The listing builds one solid part. Answer for the finished solid, in the listing's coordinates (mm). Face numbers are marked on the shaded views. A direction names the side the tool comes from. Give positions to 0.01 mm unless a question says otherwise; leave off trailing zeros. Order: outer loops, then holes, each group sorted by start corner. A loop starts at its lowest first (then second) coordinate and runs counter-clockwise, first axis right, second up.
```python
from build123d import *

# Parameters (mm, degrees)
BOSS_EXTRUDE1_DEPTH = 35
SKETCH2_R           = 2
CUT_EXTRUDE1_DEPTH  = 83.927679336
CUT_EXTRUDE2_REACH  = 64.699
SKETCH3_R           = 4


with BuildPart() as part:
    # Sketch1 → Boss-Extrude1 (new body)
    with BuildSketch(Plane(origin=(0, 0, 0), x_dir=(1, 0, 0), z_dir=(0, 1, 0))):
        with BuildLine():
            Line((-36, 30), (-36, 0))
            ThreePointArc((-36, 0), (-0.776670285, -35.991621015), (35.966487959, -1.552979031))
            Line((35.966487959, -1.552979031), (27.456115095, -1.552979031))
            ThreePointArc((27.456115095, -1.552979031), (-27.5, 0), (27.456115095, 1.552979031))
            Line((27.456115095, 1.552979031), (36, 1.552979031))
            Line((36, 1.552979031), (36, 30))
            Line((36, 30), (-36, 30))
        make_face()
    extrude(amount=BOSS_EXTRUDE1_DEPTH)

    # Sketch2 → Cut-Extrude1 (cut, through all)
    with BuildSketch(Plane(origin=(0, 0, -30), x_dir=(-1, 0, 0), z_dir=(0, 0, -1))):
        with Locations((-33, 28)):
            Circle(SKETCH2_R)
        with Locations((33, 28)):
            Circle(SKETCH2_R)
        with Locations((33, 7)):
            Circle(SKETCH2_R)
        with Locations((-33, 7)):
            Circle(SKETCH2_R)
    extrude(amount=-CUT_EXTRUDE1_DEPTH, mode=Mode.SUBTRACT)

    # Sketch3 → Cut-Extrude2 (cut, up to next)
    with BuildSketch(Plane(origin=(0, 0, 7.552979031), x_dir=(-1, 0, 0), z_dir=(0, 0, -1)), mode=Mode.PRIVATE) as cut_extrude2_sk1:
        with Locations((-33, 28)):
            Circle(SKETCH3_R)
    cut_extrude2_tool1 = extrude(cut_extrude2_sk1.sketch, amount=-CUT_EXTRUDE2_REACH, mode=Mode.PRIVATE) & part.part
    # Sketch3 → Cut-Extrude2 (cut, up to next)
    with BuildSketch(Plane(origin=(0, 0, 7.552979031), x_dir=(-1, 0, 0), z_dir=(0, 0, -1)), mode=Mode.PRIVATE) as cut_extrude2_sk2:
        with Locations((-33, 7)):
            Circle(SKETCH3_R)
    cut_extrude2_tool2 = extrude(cut_extrude2_sk2.sketch, amount=-CUT_EXTRUDE2_REACH, mode=Mode.PRIVATE) & part.part
    # Sketch3 → Cut-Extrude2 (cut, up to next)
    with BuildSketch(Plane(origin=(0, 0, 7.552979031), x_dir=(-1, 0, 0), z_dir=(0, 0, -1)), mode=Mode.PRIVATE) as cut_extrude2_sk3:
        with Locations((33, 28)):
            Circle(SKETCH3_R)
    cut_extrude2_tool3 = extrude(cut_extrude2_sk3.sketch, amount=-CUT_EXTRUDE2_REACH, mode=Mode.PRIVATE) & part.part
    # Sketch3 → Cut-Extrude2 (cut, up to next)
    with BuildSketch(Plane(origin=(0, 0, 7.552979031), x_dir=(-1, 0, 0), z_dir=(0, 0, -1)), mode=Mode.PRIVATE) as cut_extrude2_sk4:
        with Locations((33, 7)):
            Circle(SKETCH3_R)
    cut_extrude2_tool4 = extrude(cut_extrude2_sk4.sketch, amount=-CUT_EXTRUDE2_REACH, mode=Mode.PRIVATE) & part.part
    add(cut_extrude2_tool1.solids().sort_by_distance((33, 28, 7.552979))[0], mode=Mode.SUBTRACT)
    add(cut_extrude2_tool2.solids().sort_by_distance((33, 7, 7.552979))[0], mode=Mode.SUBTRACT)
    add(cut_extrude2_tool3.solids().sort_by_distance((-33, 28, 7.552979))[0], mode=Mode.SUBTRACT)
    add(cut_extrude2_tool4.solids().sort_by_distance((-33, 7, 7.552979))[0], mode=Mode.SUBTRACT)


solid = part.part
```
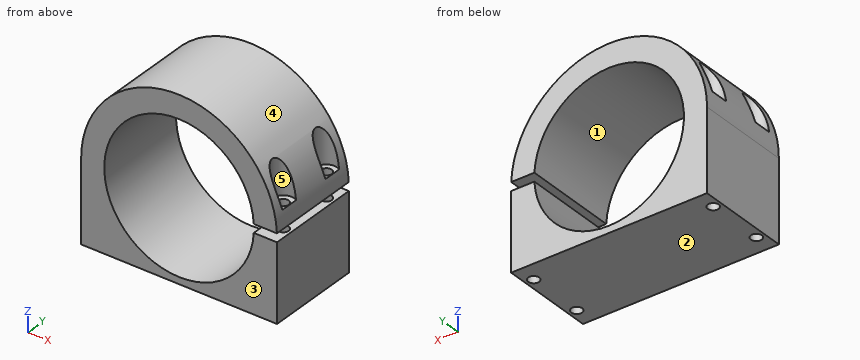
1) Find section B-B (x = 0). Write down the section's boundary in (y, z), then the cut area to 3 significant figures.
Geometry says:
outline: (0, -30) - (35, -30) - (35, -27.5) - (0, -27.5) - close; (0, 27.5) - (35, 27.5) - (35, 36) - (0, 36) - close
area: 385 mm2
2) Given P1, Ø10.5, axis at x = 33, y = 7, coming from the +Z side; P2, Ø6.5, axis at x = 33, y = 28, coming from the +Z side; P3, Ø1.9, axis at x = -33.5, y = 28, coming from the +Z side; P4, Ø3, axis at x = 15, y = 13.5, coming from the +Z side, each flat-ended and moving along its own axis, determine where each tip first touches the part or whether it passes through.
Geometry says:
P1: stops at z = 22.93
P2: stops at z = 7.55
P3: passes through
P4: stops at z = 33.37
3) Find section C-C (y = 7). Write down the section's boundary in (x, z).
Geometry says:
outline: (-36, -30) - (-35, -30) - (-35, 7.55) - (-35.2, 7.55) arc R36 ccw to (-36, 0) - close; (-31, -30) - (31, -30) - (31, -1.55) - (27.46, -1.55) arc R27.5 cw (long way) to (27.46, 1.55) - (31, 1.55) - (31, 7.55) - (29, 7.55) - (29, 21.33) arc R36 ccw to (-29, 21.33) - (-29, 7.55) - (-31, 7.55) - close; (35, -30) - (36, -30) - (36, -1.55) - (35, -1.55) - close; (35, 1.55) - (35.97, 1.55) arc R36 ccw to (35.2, 7.55) - (35, 7.55) - close
4) For a pull along Z with two mould halves and no side action, classify the marked faces 1, 2 and 3 as +Z half, -Z half, draft (parallel to the pull), parting line (faces both ways), or undercut.
Geometry says:
face 1: undercut
face 2: -Z half
face 3: draft
5) Straight lines are drawn through the part: probe 1 along Y at (x, z) = (-33, -16); probe 2 along Z at (x, y) = (1, 21); probe 3 along X at (y, z) = (7, 13.5). For each, find the intervals that lie inside material, in ascending order.
Geometry says:
probe 1: y = 0 to 5, 9 to 26, 30 to 35
probe 2: z = -30 to -27.48, 27.48 to 35.99
probe 3: x = -29 to -23.96, 23.96 to 29
6) Find section D-D (y = 22). Write down the section's boundary in (x, z).
Geometry says:
outline: (-36, -30) - (36, -30) - (36, -1.55) - (27.46, -1.55) arc R27.5 cw (long way) to (27.46, 1.55) - (35.97, 1.55) arc R36 ccw to (-36, 0) - close
7) A tool of negligible diameter and unlimited length cuts with its end or side. For the marked faces 4 and 5, from which of +Z, -Z, +X, -X, +Y, -Y can it reach the whole face along a straight path? Write none if from no direction.
Geometry says:
face 4: +Z, +Y, -Y
face 5: +Z
8) Find section A-A (z = -9.5). Write down the section's boundary in (x, y).
Geometry says:
outline: (-36, 0) - (-25.81, 0) - (-25.81, 35) - (-36, 35) - close; (25.81, 0) - (36, 0) - (36, 35) - (25.81, 35) - close; hole circle Ø4 at (-33, 7); hole circle Ø4 at (-33, 28); hole circle Ø4 at (33, 7); hole circle Ø4 at (33, 28)
